The drawing under review shows one solid part. Ordinate dimensions are in mm from its lowest x, y, z. A direction names the side the tool comes from. Give positions to 0.01 mm unless a question says otherwise; leave off trailing zeros. Write each loop counter-clockwise with the first axis right and the second up, starting at its lowest first coordinate (ties: lowest second). Pieces come first, ordered by that corner, then holes. Notation, with made-up numbers: (78, 56) -> (112, 56) arc R16 ccw to (112, 69) -> close; hole circle Ø5 at (11, 51.25). An arc over 180 degrees is marked (long way). Put each result on its own line as item: value. Start each with the question number.
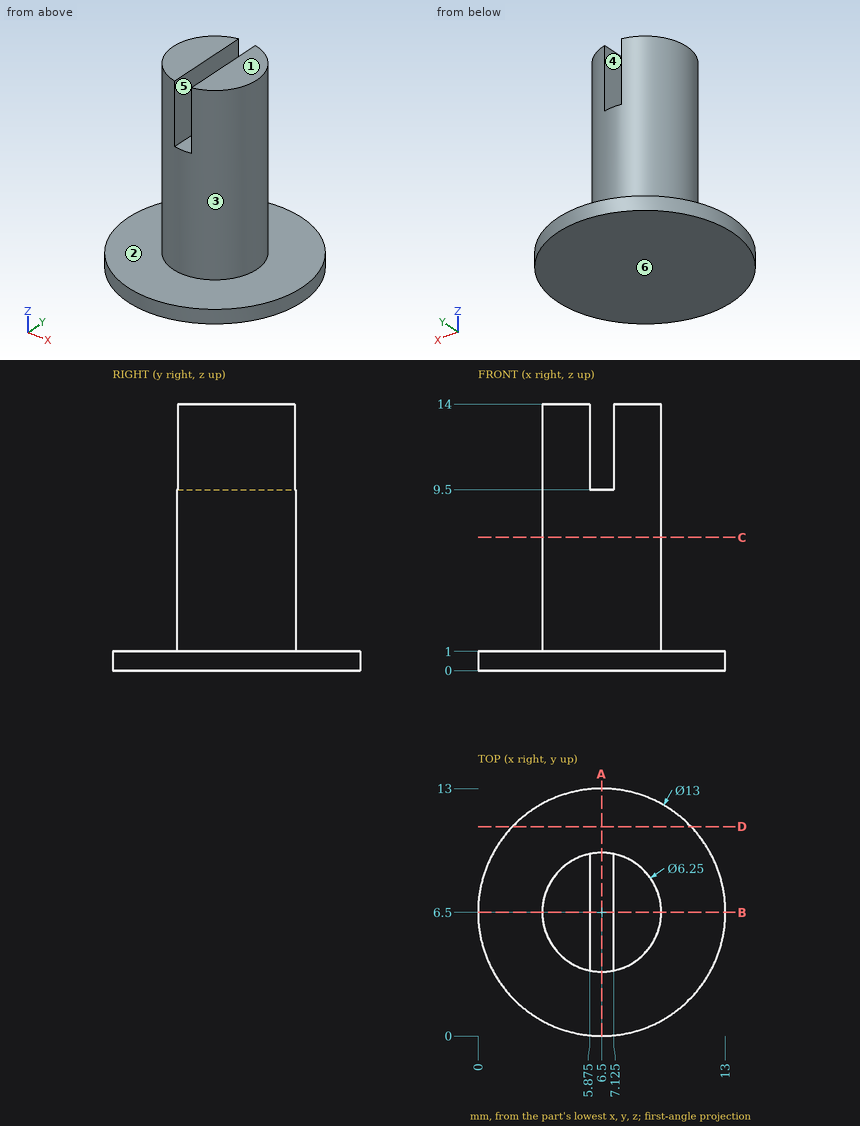
Q1. Machinability: for the marked faces 1 and 2, which of the approach directions +Z, -Z, +X, -X, +Y, -Y give a long, thin tool a straight path to every point of the face, cutting with its end or side? Answer none if there is none.
Q2. Take a section at C-C on z = 7. Give the boundary of the cut face in (x, y) (3 decimals).
Q3. Take a section at B-B on y = 6.5. Give the boundary of the cut face in (x, z) (3 decimals).
Q4. Take a section at A-A on x = 6.5. Give the boundary of the cut face in (y, z) (3 decimals).
Q5. For pin 1 (1.3 mm diameter, centred on y = 7.5, z = 12.5, fed in from +X); pin 2 (5 mm diameter, centred on y = 8, z = 12, fed in from -X) (3 decimals); pin 3 (6 mm diameter, centred on x = 10.5, z = 6, fed in from +Y); pin 4 (3 mm diameter, centred on x = 6, y = 10.5, fed in from -Z), all flat-tipped, find the tip position at first contact; note any pin that passes through.
Q6. Mouldability with a two-part tool opening along X and no side actions: class the marked faces 3, 4, 5 and 6 as +X half, -X half, draft (parallel to the pull), parting line (faces both ways), or undercut.
Q7. To check wall thickness, follow probe 1 along Z at (x, y) = (4, 8.75); probe 2 along X at (y, z) = (4.5, 11.25) (3 decimals); probe 3 along Y at (x, z) = (3.75, 10.25). State the ranges of each line that lie inside material, in increasing order. Write a range as from..to.
Q8. Take a section at D-D on y = 11. Give the boundary of the cut face in (x, z).
Result:
1. face 1: +Z, +X, -X, +Y, -Y
1. face 2: +Z
2. outline: circle Ø6.25 at (6.5, 6.5)
3. outline: (0, 0) -> (13, 0) -> (13, 1) -> (9.625, 1) -> (9.625, 14) -> (7.125, 14) -> (7.125, 9.5) -> (5.875, 9.5) -> (5.875, 14) -> (3.375, 14) -> (3.375, 1) -> (0, 1) -> close
4. outline: (0, 0) -> (13, 0) -> (13, 1) -> (9.625, 1) -> (9.625, 9.5) -> (3.375, 9.5) -> (3.375, 1) -> (0, 1) -> close
5. pin 1: stops at x = 9.61
5. pin 2: stops at x = 3.375
5. pin 3: stops at y = 9.46
5. pin 4: stops at z = 0
6. face 3: parting line
6. face 4: undercut
6. face 5: undercut
6. face 6: draft
7. probe 1: z = 0..1
7. probe 2: x = 4.099..5.875, 7.125..8.901
7. probe 3: y = 5.02..7.98
8. outline: (1.81, 0) -> (11.19, 0) -> (11.19, 1) -> (1.81, 1) -> close
